Work out the finished part from the listing and answer in its coordinate system (mm). A direction names the side the tool comes from. Give positions to 0.01 mm unless a question says otherwise; leave off trailing zeros. Loops run counter-clockwise (first coordinate to the right, second up) from the corner with the lowest first, then second, coordinate; pieces in that order, holes last. Notation, with made-up numbers: M -19.75,10.5 L -15.75,10.5 A31 ccw -15.75,37.5 Z; hole C 49.5,37.25 d2. An arc over 180 degrees is marked long. Use a Markdown table: item, result.
```python
from build123d import *

# Parameters (mm, degrees)
BOSS_EXTRU_1_DEPTH      = 308
ESQUISSE2_W             = 8
ESQUISSE2_H             = 100
ESQUISSE2_H_2           = 55
ENL_V_MAT_EXTRU_1_DEPTH = 8
ESQUISSE3_W             = 172
ESQUISSE3_H             = 280.536291501
ENL_V_MAT_EXTRU_2_DEPTH = 532
ESQUISSE4_R             = 1.6
ESQUISSE4_W             = 172
ESQUISSE4_H             = 279.620784643
ENL_V_MAT_EXTRU_3_DEPTH = 8
ESQUISSE5_W             = 182
ESQUISSE5_H             = 290.536291501
ENL_V_MAT_EXTRU_4_DEPTH = 3
ESQUISSE6_W             = 182
ESQUISSE6_H             = 290
ENL_V_MAT_EXTRU_5_DEPTH = 3
ESQUISSE7_R             = 4
ENL_V_MAT_EXTRU_6_DEPTH = 5.3
ESQUISSE8_W             = 8.5
ESQUISSE8_H             = 406.733495256
ENL_V_MAT_EXTRU_7_DEPTH = 4
ESQUISSE9_W             = 8.5
ESQUISSE9_H             = 359.311541269
ENL_V_MAT_EXTRU_8_DEPTH = 4


with BuildPart() as part:
    # Esquisse1 → Boss.-Extru.1 (new body)
    with BuildSketch(Plane.XY):
        Polygon((-49.970813456, -41.917379116), (-57.970813456, -41.917379116), (-57.970813456, 358.618912385), (-313.627667703, 614.275766632), (-307.970813453, 619.932620882), (-49.970813456, 361.932620884), align=None)
    extrude(amount=BOSS_EXTRU_1_DEPTH)

    # Esquisse2 → Enlèv. mat.-Extru.1 (cut)
    with BuildSketch(Plane.XY.offset(308)):
        with Locations((-53.970813456, 8.082620884)):
            Rectangle(ESQUISSE2_W, ESQUISSE2_H)
        Polygon((-271.201260832, 571.849359761), (-265.544406582, 577.506214011), (-307.970813453, 619.932620882), (-313.627667703, 614.275766632), align=None)
        with Locations((-53.970813456, 140.582620884)):
            Rectangle(ESQUISSE2_W, ESQUISSE2_H_2)
        with Locations((-53.970813456, 250.582620884)):
            Rectangle(ESQUISSE2_W, ESQUISSE2_H_2)
        Polygon((-232.310387866, 532.958486796), (-226.653533617, 538.615341045), (-187.762660652, 499.72446808), (-193.419514901, 494.067613831), align=None)
        Polygon((-154.528641936, 455.176740865), (-148.871787686, 460.833595115), (-109.980914721, 421.94272215), (-115.637768971, 416.2858679), align=None)
        Polygon((-76.746896005, 377.394994935), (-71.090041756, 383.051849184), (-49.970813456, 361.932620884), (-49.970813456, 333.082620884), (-57.970813456, 333.082620884), (-57.970813456, 358.618912385), align=None)
    extrude(amount=-ENL_V_MAT_EXTRU_1_DEPTH, mode=Mode.SUBTRACT)

    # Esquisse3 → Enlèv. mat.-Extru.2 (cut)
    with BuildSketch(Plane.ZY.offset(57.970813456)):
        with Locations((194, 198.350766635)):
            Rectangle(ESQUISSE3_W, ESQUISSE3_H)
    extrude(amount=-ENL_V_MAT_EXTRU_2_DEPTH, mode=Mode.SUBTRACT)

    # Esquisse4 → Enlèv. mat.-Extru.3 (cut)
    with BuildSketch(Plane(origin=(155.980903714, 155.980903714, 0), x_dir=(0, 0, -1), z_dir=(0.707106781186556, 0.7071067811865391, 0))):
        with Locations(Location((-150, 652.126810705, 0), (0, 0, 90))):
            Circle(ESQUISSE4_R)
        with BuildLine():
            Line((-202.2627417, 648.126810705), (-300, 648.126810705))
            Line((-300, 648.126810705), (-300, 656.126810705))
            Line((-300, 656.126810705), (-200, 656.126810705))
            Line((-200, 656.126810705), (-200, 650.389552405))
            ThreePointArc((-200, 650.389552405), (-200, 648.126810705), (-202.2627417, 648.126810705))
        make_face()
        with BuildLine():
            Line((-100, 656.126810705), (-100, 650.389552405))
            ThreePointArc((-100, 650.389552405), (-100, 648.126810705), (-97.7372583, 648.126810705))
            Line((-97.7372583, 648.126810705), (0, 648.126810705))
            Line((0, 648.126810705), (0, 656.126810705))
            Line((0, 656.126810705), (-100, 656.126810705))
        make_face()
        with Locations((-194, 455.937203027)):
            Rectangle(ESQUISSE4_W, ESQUISSE4_H)
    extrude(amount=-ENL_V_MAT_EXTRU_3_DEPTH, mode=Mode.SUBTRACT)

    # Esquisse5 → Enlèv. mat.-Extru.4 (cut)
    with BuildSketch(Plane.ZY.offset(57.970813456)):
        with Locations((194, 198.350766635)):
            Rectangle(ESQUISSE5_W, ESQUISSE5_H)
    extrude(amount=-ENL_V_MAT_EXTRU_4_DEPTH, mode=Mode.SUBTRACT)

    # Esquisse6 → Enlèv. mat.-Extru.5 (cut)
    with BuildSketch(Plane(origin=(150.324049465, 150.324049465, 0), x_dir=(0, 0, 1), z_dir=(-0.707106781186556, -0.7071067811865391, 0))):
        with Locations((194, 455.747595348)):
            Rectangle(ESQUISSE6_W, ESQUISSE6_H)
    extrude(amount=-ENL_V_MAT_EXTRU_5_DEPTH, mode=Mode.SUBTRACT)

    # Esquisse7 → Enlèv. mat.-Extru.6 (cut)
    with BuildSketch(Plane.ZY.offset(57.970813456)):
        with Locations((20, -21.917379116)):
            Circle(ESQUISSE7_R)
    extrude(amount=-ENL_V_MAT_EXTRU_6_DEPTH, mode=Mode.SUBTRACT)

    # Esquisse8 → Enlèv. mat.-Extru.7 (cut)
    with BuildSketch(Plane.ZY.offset(57.970813456)):
        with Locations((94.25, 157.026144561)):
            Rectangle(ESQUISSE8_W, ESQUISSE8_H)
    extrude(amount=-ENL_V_MAT_EXTRU_7_DEPTH, mode=Mode.SUBTRACT)

    # Esquisse9 → Enlèv. mat.-Extru.8 (cut)
    with BuildSketch(Plane(origin=(150.324049465, 150.324049465, 0), x_dir=(0, 0, 1), z_dir=(-0.7071067811865559, -0.7071067811865391, 0))):
        with Locations((94.25, 472.802749855)):
            Rectangle(ESQUISSE9_W, ESQUISSE9_H)
    extrude(amount=-ENL_V_MAT_EXTRU_8_DEPTH, mode=Mode.SUBTRACT)


solid = part.part
```
(1) Which of the six approach directions +Z, -Z, +X, -X, +Y, -Y give full straight-line access (tool end or side, diameter ignored) to faces 4 (the flat face through (-54.971, 242, 281)), 5 (the flat face through (-223.08, 523.73, 288.11))?
Entries:
| item | result |
|---|---|
| face 4 | -X |
| face 5 | +Z, -Z, -X, -Y |
(2) A cutting plane is placed at C-C (x = -173.5). Write down the section's boundary in (y, z).
Entries:
| item | result |
|---|---|
| outline | M 474.15,0 L 485.46,0 L 485.46,108 L 478.39,108 L 478.39,103 L 474.15,103 L 474.15,98.5 L 479.8,98.5 L 479.8,90 L 474.15,90 Z; M 474.15,285 L 478.39,285 L 478.39,280 L 485.46,280 L 485.46,308 L 474.15,308 Z |
(3) Consider probe 1 along Y at (x, z) = (-53.8, 20); probe 2 along Y at (x, z) = (-54.6, 20); probe 3 along X at (y, z) = (180, 82). Determine where each line is inside the solid, lowest interval first. Write a range as [from, to].
Entries:
| item | result |
|---|---|
| probe 1 | y = [-41.92, -25.92], [-17.92, 365.76] |
| probe 2 | y = [-41.92, -25.92], [-17.92, 366.56] |
| probe 3 | x = [-57.97, -49.97] |
(4) A cutting plane is placed at B-B (y = 409.5). Write down the section's boundary in (x, z).
Entries:
| item | result |
|---|---|
| outline | M -108.85,0 L -97.54,0 L -97.54,108 L -104.61,108 L -104.61,103 L -108.85,103 L -108.85,98.5 L -103.2,98.5 L -103.2,90 L -108.85,90 Z; M -108.85,285 L -104.61,285 L -104.61,280 L -97.54,280 L -97.54,308 L -108.85,308 Z |
(5) The mould has two halves that part along Z. Classify faces 1 (the flat face through (-169, 472, 103)), 2 (the flat face through (-57.971, 39, 211)), 3 (the flat face through (-249, 555, 308)): released by +Z, released by -Z, zero draft, split by the parting line, or undercut.
Entries:
| item | result |
|---|---|
| face 1 | undercut |
| face 2 | zero draft |
| face 3 | released by +Z |
(6) A cutting plane is placed at D-D (x = -283). Write down the section's boundary in (y, z), and give its area (3 significant figures).
Entries:
| item | result |
|---|---|
| outline | M 583.65,0 L 594.96,0 L 594.96,300 L 583.65,300 L 583.65,98.5 L 589.3,98.5 L 589.3,90 L 583.65,90 Z |
| area | 3,350 mm² |
(7) Given P1, Ø4, axis at x = -53.5, z = 304.5, coming from the +Y side; P2, Ø2.5, axis at y = 227.5, z = 94, coming from the -X side; P3, Ø1, axis at x = -224.5, z = 59.5, coming from the +Y side; P4, Ø3.5, axis at x = -55.5, y = 225, coming from the -Z side, each flat-ended and moving along its own axis, determine where each tip first touches the part or whether it passes through.
Entries:
| item | result |
|---|---|
| P1 | stops at y = 333.08 |
| P2 | stops at x = -53.97 |
| P3 | stops at y = 536.96 |
| P4 | stops at z = 0 |
(8) A cutting plane is placed at A-A (z = 130). Write down the section's boundary in (x, y).
Entries:
| item | result |
|---|---|
| outline | M -313.63,614.28 L -274.47,575.12 L -272.35,577.24 L -268.81,573.7 L -265.28,577.24 L -307.97,619.93 Z; M -71.09,375.98 L -67.29,372.18 L -69.41,370.06 L -57.97,358.62 L -57.97,343.62 L -54.97,343.62 L -54.97,338.62 L -49.97,338.62 L -49.97,361.93 L -67.55,379.52 Z; M -57.97,-41.92 L -49.97,-41.92 L -49.97,58.08 L -54.97,58.08 L -54.97,53.08 L -57.97,53.08 Z |
